Geometry check sheet. Reference: the model listing, model coordinates, mm. Round coordinates to 2 decimals unless told otherwise and drop trailing zeros. Loops run counter-clockwise (first coordinate to the right, second up) from the corner with the lowest first, then second, coordinate; pieces in that order, holes last. Notation, with made-up numbers: M -39,-7 L -18,-7 A11 ccw -18,13 Z; hole C 2.5,28.25 d3. An arc over 180 degrees is marked long. Write item = value, one per line.
Autodesk Inventor part; units mm, degrees
ref_plane "YZ Plane" through (0, 0, 0) normal (1, 0, 0) x (0, 1, 0)
ref_plane "XZ Plane" through (0, 0, 0) normal (0, 1, 0) x (-1, 0, 0)
ref_plane "XY Plane" through (0, 0, 0) normal (0, 0, 1) x (1, 0, 0)
sketch "Sketch1" plane through (0, 0, 0) normal (1, 0, 0) x (0, 1, 0)
  line L0 (0, 0) -> (0, -10) construction
  line L1 (0, -10) -> (0, -50) construction
  circle A0 centre (0, -10) radius 1.905
  circle A1 centre (0, -50) radius 1.905
  line L2 (10, 0) -> (10, -59)
  line L3 (10, -59) -> (0, -59)
  line L4 (0, -59) -> (-10, -59)
  line L5 (-10, -59) -> (-10, 0)
  line L6 (0, 0) -> (10, 0)
  line L7 (0, 0) -> (-10, 0)
  line L8 (0, -50) -> (0, -59) construction
  circle A2 centre (0, 40) radius 25
  line L9 (10, 0) -> (10, 10)
  line L10 (10, 10) -> (-10, 10)
  line L11 (-10, 10) -> (-10, 0)
  arc A3 (22.8049, 29.7561) -> (10, -30) centre (155.8333, -30) ccw
  arc A4 (-10, -30) -> (-22.8049, 29.7561) centre (-155.8333, -30) ccw
  line L12 (0, -30) -> (21, -30) construction
  line L13 (0, -30) -> (-21, -30) construction
  circle A5 centre (21, -30) radius 3.5
  circle A6 centre (-21, -30) radius 3.5
  circle A7 centre (21, -30) radius 10
  circle A8 centre (-21, -30) radius 10
  circle A9 centre (21, -30) radius 6.5
  circle A10 centre (-21, -30) radius 6.5
  line L14 (-10, -59) -> (-25, -59)
  line L15 (10, -59) -> (25, -59)
  arc A11 (-28.9586, -23.9452) -> (-22.8049, 29.7561) centre (-71.0556, 8.082) ccw
  arc A12 (22.8049, 29.7561) -> (28.9586, -23.9452) centre (71.0556, 8.082) ccw
  line L16 (0, 0) -> (15, 0)
  line L17 (10, 0) -> (25, 0)
  line L18 (25, -59) -> (25, -50.3)
  arc A13 (29.3932, -35.4364) -> (25, -50.3) centre (52.3408, -50.3) ccw
  line L19 (25, 0) -> (25, -8.7)
  arc A14 (25, -8.7) -> (29.5297, -24.7804) centre (55.8075, -8.7) ccw
  line L20 (-10, 0) -> (-25, 0)
  line L21 (-25, -59) -> (-25, -50.3)
  arc A15 (-25, -50.3) -> (-29.3932, -35.4364) centre (-52.3408, -50.3) ccw
  line L22 (-25, 0) -> (-25, -8.7)
  arc A16 (-29.5297, -24.7804) -> (-25, -8.7) centre (-55.8075, -8.7) ccw
  circle A17 centre (0, -50) radius 4
  circle A18 centre (0, -10) radius 4
  circle A19 centre (0, 40) radius 7.235
  circle A20 centre (0, 40) radius 5.08
  point P0 (-10, -30)
  point P1 (10, -30)
  point P2 (23.8246, -39.5928)
  point P3 (10, -63.336)
  point P4 (-30.2308, -33.8462)
  point P5 (28.9586, -23.9452)
  point P6 (22.8049, 29.7561)
  point P7 (30.2308, -26.1538)
  point P8 (18.7815, 0)
  point P9 (-18.7815, 0)
  point P10 (-13.1191, 0)
  point P11 (-29.3932, -35.4364)
  dimension "d0" = 3.81
  dimension "d1" = 3.81
  dimension "d2" = 40
  dimension "d3" = 10
  dimension "d5" = 9
  dimension "d7" = 10
  dimension "d8" = 10
  dimension "d9" = 50
  dimension "d12" = 30
  dimension "d13" = 10
  dimension "d14" = 20
  dimension "d30" = 21
  dimension "d31" = 7
  dimension "d32" = 7
  dimension "d33" = 20
  dimension "d34" = 20
  dimension "d38" = 3
  dimension "d48" = 15
  dimension "d55" = 15
  dimension "d56" = 8.7
  dimension "d57" = 8.7
  dimension "d58" = 15
  dimension "d134" = 8
  dimension "d135" = 8
  dimension "d138" = 14.47
  dimension "d157" = 10.16
extrude "Extrusion1" add sketch "Sketch1" along normal blind 5 contours L16 A3 L2 | L2 L3 L4 L5 L7 L6 | L6 L7 L11 L10 L9 | L9 L10 L11 L20 A4 A2 A3 L16 | A3 L16 L17 A12 A7 A13 L18 L15 L2 | A3 A12 L17 L16 | L5 A4 L20 | A2 | L5 L14 L21 A15 A8 A11 L20 A4 | L20 A11 A4 | L17 L19 A14 A7 A12 | A11 A8 A16 L22 L20 | A7 | A8 | A5 | A6 | A9 | A10 | A17 | A18 | A19 | A20
fillet "Face Fillet1" radius 5 1 edges at (2.5, -18.7815, 0)
fillet "Face Fillet2" radius 5 1 edges at (2.5, 18.7815, 0)
extrude "Extrusion16" cut sketch "Sketch1" along normal up to surface (5 mm away) contours A20
extrude "Extrusion17" cut sketch "Sketch1" along normal blind 2 from surface at 0 contours A19 | A20
extrude "Extrusion11" cut sketch "Sketch1" against normal blind 2.5 from surface at 5 contours A17 | A18
extrude "Extrusion19" add sketch "Sketch1" against normal blind 15 contours A5 | A6
extrude "Extrusion20" add sketch "Sketch1" against normal blind 5 contours A9 | A10
fillet "Fillet4" radius 2 2 edges at (-15, 17.5, -30) (-15, -24.5, -30)
chamfer "Chamfer2" distance 2 angle 45 7 edges at (5, 0, 65) (5, -19.0046, 17.4944) (5, -19.8398, 1.3525) (5, -24.1298, 0) (5, 19.0046, 17.4944) (5, 19.8398, 1.3525) (5, 24.1298, 0)
sketch "Sketch15" plane through (0, 0, 0) normal (-1, 0, 0) x (0, 0, 1)
  line L0 (0, 25) -> (0, 23.2597)
  line L1 (0, 25) -> (-8, 25)
  line L2 (-8, 25) -> (-8, 22)
  line L3 (-8, 22) -> (0, 22)
  line L4 (0, 22) -> (0, 25)
  point P0 (0, 0)
  dimension "d175" = 8
  dimension "d176" = 3
extrude "Extrusion21" add sketch "Sketch15" along normal blind 8
sketch "Sketch16" plane through (0, 25, -8.7) normal (0, 1, 0) x (1, 0, 0)
  circle A0 centre (-4, -4.7) radius 1.905
  line L0 (-8, -8.7) -> (-8, -0.7)
  line L1 (-8, -8.7) -> (3, -8.7)
  point P0 (0, -8.7)
  dimension "d179" = 3.81
  dimension "d180" = 4
  dimension "d181" = 4
extrude "Extrusion22" cut sketch "Sketch16" against normal up to surface (3 mm away)
mirror "Mirror2" about plane through (0, 0, 0) normal (0, 1, 0) of "Extrusion22", "Extrusion21"
equation "\"d0\" = M4_HOLE_D"
equation "\"d1\" = d0"
equation "\"d14\" = 0.5 * d2"
equation "\"d32\" = d31"
equation "\"d34\" = d33"
equation "\"M4_HOLE_D\" = 3.81"
equation "\"M3_HOLE_D\" = 2.54"
equation "\"d88\" = 3"
properties part number "bldc_arm" material "ABS Plastic"
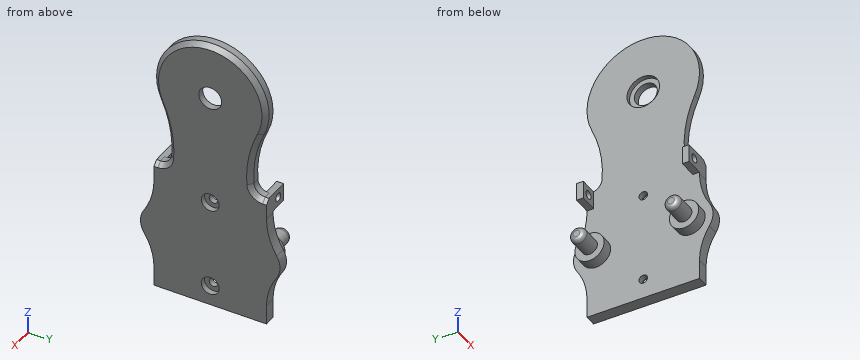
(1) Depth check by flat-ended pin: pin 1 Ø16.5 at (y, z) = (0, 40) entering from -X; pin 2 Ø9 at (x, z) = (-4, -3) entering from +Y; pin 3 Ø12 at (x, z) = (-10, -36.5) entering from +Y; pin 4 Ø6 at (x, y) = (-4.5, -7) entering from -Z. Enter the tip coordinate at first touch or a pass-through.
Result set:
pin_1 = 0
pin_2 = 25
pin_3 = 26.67
pin_4 = through
(2) Sectioned sample at C-C on z = -43. Record the cut outline in (x, y).
Result set:
outline = M 0,-25.99 L 5,-25.99 L 5,25.99 L 0,25.99 Z
(3) Sectioned sample at A-A on z = -4. Record the cut outline in (x, y) (3 decimals), then the cut area to 3 significant figures.
Result set:
outline = M -8,-25 L -5.905,-25 L -5.905,-22 L -8,-22 Z; M -8,22 L -5.905,22 L -5.905,25 L -8,25 Z; M -2.095,-25 L 5,-25 L 5,25 L -2.095,25 L -2.095,22 L 0,22 L 0,-22 L -2.095,-22 Z
area = 275 mm2
(4) Sectioned sample at B-B on x = -9.5. Record the cut outline in (y, z), then the cut area to 3 significant figures.
Result set:
outline = C -21,-30 d7; C 21,-30 d7
area = 77.0 mm2
(5) Material ranges on line 1 along Z through (x, y) = (1.65, 0) (3 decimals); line 2 along X through (y, z) = (-23.25, -4) (3 decimals); line 3 along Z through (x, y) = (3.6, 0), recorded low to high. Write a range as from..to.
Result set:
line_1 = -59..-51.905, -48.095..-11.905, -8.095..32.765, 47.235..65
line_2 = -8..-5.905, -2.095..5
line_3 = -59..-54, -46..-14, -6..34.92, 45.08..64.4
